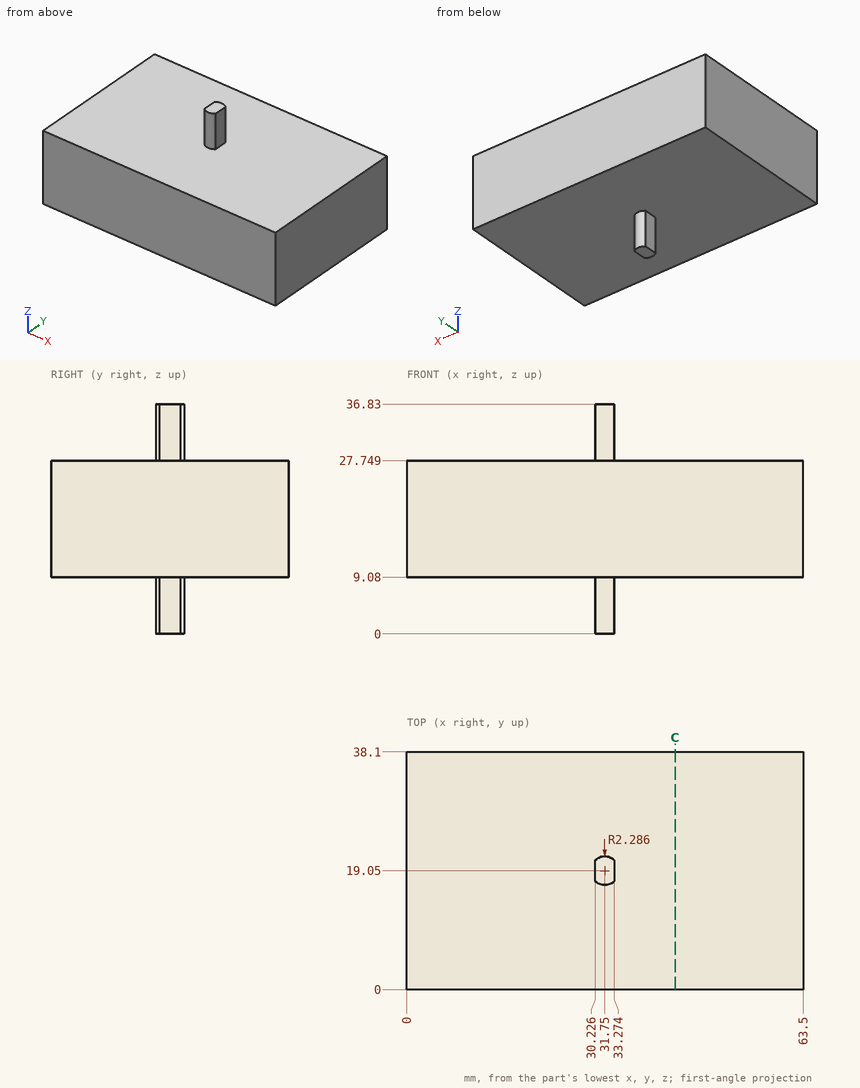
For this review, use the dimensioned drawing (mm, ordinates from the lowest corner) and the shaded views. Round coordinates to 2 decimals unless told otherwise and drop trailing zeros. Write each loop counter-clockwise with the first axis right and the second up, starting at its lowest first coordinate (ties: lowest second). Pieces come first, ordered by that corner, then holes. Notation, with made-up numbers: (20.25, 84.5) -> (28.25, 84.5) arc R4 cw to (28.25, 89.5) -> close; hole circle Ø10 at (48, -5). An arc over 180 degrees is marked (long way). Use CSV: the item, a comma, the result in double quotes.
Q1. Consider section C-C (x = 43). Give the boundary of the cut face in (y, z).
Checks:
outline,"(0, 9.08) -> (38.1, 9.08) -> (38.1, 27.75) -> (0, 27.75) -> close"
Q2. For pin 1 Ø12 at (x, y) = (51, 23) entering from -Z; pin 2 Ø4 at (x, y) = (53.5, 20.5) entering from +Z; pin 3 Ø2.5 at (y, z) = (18.5, 31) entering from +X, all flat-tipped, find the tip position at first contact; note any pin that passes through.
Checks:
pin 1,"z = 9.08"
pin 2,"z = 27.75"
pin 3,"x = 33.27"
Q3. To check wall thickness, follow probe 1 along X at (y, z) = (18, 30) (1 decimal); probe 2 along Z at (x, y) = (24, 11). State the ranges of each line that lie inside material, in increasing order. Write a range as [from, to].
Checks:
probe 1,"[30.2, 33.3]"
probe 2,"[9.08, 27.75]"
